from build123d import *

# Parameters (mm, degrees)
SKETCH_1_R      = 5
EXTRUDE_1_DEPTH = 150
SKETCH_2_R      = 10
EXTRUDE_2_DEPTH = 5
CHAMFER_1_SIZE  = 3


with BuildPart() as part:
    # 草图1 → 凸台-拉伸1 (new body)
    with BuildSketch(Plane(origin=(0, 0, 0), x_dir=(0, 0, -1), z_dir=(1, 0, 0))):
        Circle(SKETCH_1_R)
    extrude(amount=EXTRUDE_1_DEPTH)

    # 草图2 → 凸台-拉伸2 (add)
    with BuildSketch(Plane.ZY):
        Circle(SKETCH_2_R)
    extrude(amount=EXTRUDE_2_DEPTH)

    # 倒角1
    chamfer_1_edges = [part.edges().sort_by_distance(p)[0] for p in [
        (0, 0, 5),
    ]]
    chamfer(chamfer_1_edges, length=CHAMFER_1_SIZE)


solid = part.part
Could you check a few things on this model? Use its own coordinates, in mm. A direction names the side the tool comes from. Coordinates: 2 decimals unless noted, no trailing zeros. Order: outer loops, then holes, each group sorted by start corner. A loop starts at its lowest first (then second) coordinate and runs counter-clockwise, first axis right, second up. Notation, with made-up numbers: (44, 55.5) -> (80, 55.5) arc R30 cw to (80, 85.5) -> close; hole circle Ø4 at (69, 22.5). An arc over 180 degrees is marked (long way). One line per question, with ' | ' between items.
Q1. On a 3-axis mill with a long thin cutter (end or side, diameter ignored), from which of +Z, -Z, +X, -X, +Y, -Y can I reach the whole of each face in a straight line? I mean faces 1 (the face through (-5, 0, 0)), 2 (the face through (0, 8.2, 0)). Say none if no direction works.
Return value:
face 1: +Z, -Z, -X, +Y, -Y | face 2: +X
Q2. Imagine slicing it at A-A on y = 0. Please give me the cut outline in (x, z), and give its area (3 significant figures).
Return value:
outline: (-5, -10) -> (0, -10) -> (0, -8) -> (3, -5) -> (150, -5) -> (150, 5) -> (3, 5) -> (0, 8) -> (0, 10) -> (-5, 10) -> close | area: 1,610 mm²
Q3. If I drill on L1, parallel to Z at x = 85, y = -0.5; L2, parallel to X at y = -7.75, z = -3.25; L3, parallel to Y at x = 5.5, z = 0.25, over which ranges is the centre line in solid material (lowest first)?
Return value:
L1: -4.97 to 4.97 | L2: -5 to 0 | L3: -4.99 to 4.99
Q4. Imagine slicing it at C-C on x = 75. Please give me the cut outline in (y, z).
Return value:
outline: circle Ø10 at (0, 0)
Q5. I'm going to push flat-ended pins straight in: P1, Ø12, axis at x = 81, y = -6, coming from the +Z side; P2, Ø3, axis at x = 73, z = -4.5, coming from the -Y side; P3, Ø3, axis at x = 82.5, y = -5.5, coming from the -Z side. Where does each tip first touch, or does it pass through?
Return value:
P1: z = 5 | P2: y = -4 | P3: z = -3
